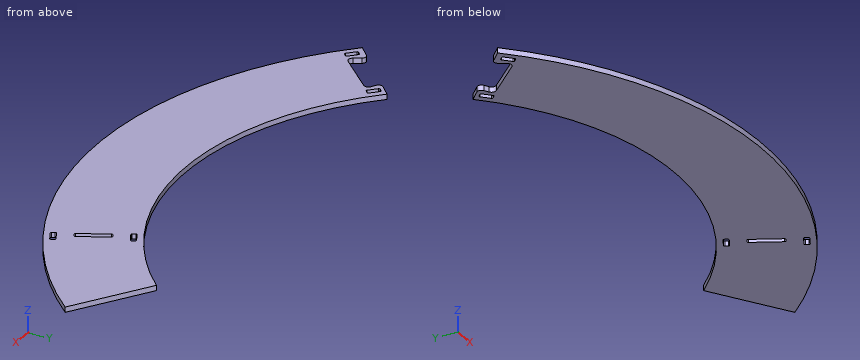
Autodesk Inventor part; units mm, degrees
ref_plane "YZ Plane" through (0, 0, 0) normal (1, 0, 0) x (0, 1, 0)
ref_plane "XZ Plane" through (0, 0, 0) normal (0, 1, 0) x (-1, 0, 0)
ref_plane "XY Plane" through (0, 0, 0) normal (0, 0, 1) x (1, 0, 0)
sketch "CONTOURS" plane through (0, 0, 0) normal (0, 0, 1) x (1, 0, 0)
  arc A0 (18.8569, 427.8827) -> (1891.4893, 468.7097) centre (936.3152, 1313.2613) ccw
  line L0 (18.8569, 427.8827) -> (54.648, 462.3952)
  arc A1 (77.2131, 459.3056) -> (54.648, 462.3952) centre (64.7129, 451.9575) ccw
  line L1 (77.2131, 459.3056) -> (90.7845, 436.2188)
  arc A2 (90.7845, 436.2188) -> (115.4755, 433.495) centre (104.1468, 444.0737) ccw
  line L2 (115.4755, 433.495) -> (224.0619, 549.7797)
  arc A3 (224.0619, 549.7797) -> (220.3778, 573.8421) centre (212.7332, 560.3584) ccw
  line L3 (220.3778, 573.8421) -> (205.6826, 582.1735)
  arc A4 (202.7691, 605.2251) -> (205.6826, 582.1735) centre (212.834, 594.7873) ccw
  line L4 (202.7691, 605.2251) -> (237.5129, 638.7277)
  arc A5 (237.5129, 638.7277) -> (1635.1174, 638.7277) centre (936.3152, 1313.2613) ccw
  line L5 (1635.1174, 638.7277) -> (1891.4893, 468.7097)
sketch "HOLES" plane through (0, 0, 0) normal (0, 0, 1) x (1, 0, 0)
  arc A0 (75.3736, 400.9492) -> (81.0303, 400.9936) centre (78.1798, 403.7997) ccw
  line L0 (75.3736, 400.9492) -> (49.7191, 426.2049)
  arc A1 (49.6748, 431.8616) -> (49.7191, 426.2049) centre (52.5253, 429.0554) ccw
  line L1 (49.6748, 431.8616) -> (57.3918, 439.7004)
  arc A2 (63.0485, 439.7447) -> (57.3918, 439.7004) centre (60.2423, 436.8942) ccw
  line L2 (63.0485, 439.7447) -> (88.703, 414.4891)
  arc A3 (88.7473, 408.8324) -> (88.703, 414.4891) centre (85.8968, 411.6386) ccw
  line L3 (1537.9287, 212.5375) -> (1505.9814, 195.9431)
  arc A4 (1500.5879, 197.6489) -> (1505.9814, 195.9431) centre (1504.1376, 199.4928) ccw
  line L4 (1500.5879, 197.6489) -> (1495.5174, 207.4106)
  arc A5 (1497.2233, 212.8041) -> (1495.5174, 207.4106) centre (1499.0671, 209.2544) ccw
  line L5 (1497.2233, 212.8041) -> (1529.1705, 229.3985)
  arc A6 (1534.564, 227.6927) -> (1529.1705, 229.3985) centre (1531.0143, 225.8489) ccw
  line L6 (1534.564, 227.6927) -> (1539.6345, 217.931)
  arc A7 (1537.9287, 212.5375) -> (1539.6345, 217.931) centre (1536.0848, 216.0872) ccw
  line L7 (1485.873, 267.1962) -> (1476.1114, 262.1257)
  arc A8 (1470.7179, 263.8316) -> (1476.1114, 262.1257) centre (1474.2676, 265.6754) ccw
  line L8 (1470.7179, 263.8316) -> (1420.4735, 360.5606)
  arc A9 (1422.1794, 365.9541) -> (1420.4735, 360.5606) centre (1424.0232, 362.4044) ccw
  line L9 (1422.1794, 365.9541) -> (1431.9411, 371.0247)
  arc A10 (1437.3346, 369.3188) -> (1431.9411, 371.0247) centre (1433.7849, 367.475) ccw
  line L10 (1437.3346, 369.3188) -> (1487.5789, 272.5898)
  arc A11 (1485.873, 267.1962) -> (1487.5789, 272.5898) centre (1484.0292, 270.7459) ccw
  line L11 (1388.5747, 413.294) -> (1383.5041, 423.0556)
  arc A12 (1385.21, 428.4491) -> (1383.5041, 423.0556) centre (1387.0538, 424.8994) ccw
  line L12 (1385.21, 428.4491) -> (1417.1572, 445.0436)
  arc A13 (1422.5507, 443.3377) -> (1417.1572, 445.0436) centre (1419.001, 441.4939) ccw
  line L13 (1422.5507, 443.3377) -> (1427.6212, 433.5761)
  arc A14 (1425.9154, 428.1826) -> (1427.6212, 433.5761) centre (1424.0716, 431.7322) ccw
  line L14 (1425.9154, 428.1826) -> (1393.9682, 411.5881)
  arc A15 (1388.5747, 413.294) -> (1393.9682, 411.5881) centre (1392.1243, 415.1378) ccw
  line L15 (220.1514, 605.0305) -> (227.8684, 612.8694)
  arc A16 (233.5251, 612.9137) -> (227.8684, 612.8694) centre (230.7189, 610.0632) ccw
  line L16 (233.5251, 612.9137) -> (259.1796, 587.658)
  arc A17 (259.2239, 582.0014) -> (259.1796, 587.658) centre (256.3734, 584.8075) ccw
  line L17 (259.2239, 582.0014) -> (251.5069, 574.1625)
  arc A18 (245.8502, 574.1182) -> (251.5069, 574.1625) centre (248.6564, 576.9687) ccw
  line L18 (245.8502, 574.1182) -> (220.1957, 599.3738)
  arc A19 (220.1514, 605.0305) -> (220.1957, 599.3738) centre (223.0019, 602.2243) ccw
  line L19 (543.0858, 821.5545) -> (547.6833, 831.5476)
  arc A20 (547.6833, 831.5476) -> (545.7213, 836.8533) centre (544.0494, 833.2195) ccw
  line L20 (545.7213, 836.8533) -> (513.0165, 851.8999)
  arc A21 (513.0165, 851.8999) -> (507.7108, 849.9379) centre (511.3447, 848.266) ccw
  line L21 (507.7108, 849.9379) -> (503.1133, 839.9447)
  arc A22 (503.1133, 839.9447) -> (505.0753, 834.639) centre (506.7471, 838.2729) ccw
  line L22 (505.0753, 834.639) -> (537.7801, 819.5925)
  arc A23 (537.7801, 819.5925) -> (543.0858, 821.5545) centre (539.4519, 823.2264) ccw
  line L23 (481.0423, 782.4016) -> (435.4847, 683.3788)
  arc A24 (435.4847, 683.3788) -> (437.4468, 678.0731) centre (439.1186, 681.7069) ccw
  line L24 (437.4468, 678.0731) -> (447.4399, 673.4755)
  arc A25 (447.4399, 673.4755) -> (452.7456, 675.4376) centre (449.1117, 677.1094) ccw
  line L25 (452.7456, 675.4376) -> (498.3031, 774.4603)
  arc A26 (498.3031, 774.4603) -> (496.3411, 779.766) centre (494.6693, 776.1322) ccw
  line L26 (496.3411, 779.766) -> (486.348, 784.3636)
  arc A27 (486.348, 784.3636) -> (481.0423, 782.4016) centre (484.6762, 780.7297) ccw
  line L27 (446.1185, 610.7891) -> (441.521, 600.7959)
  arc A28 (436.2153, 598.8339) -> (441.521, 600.7959) centre (437.8871, 602.4678) ccw
  line L28 (436.2153, 598.8339) -> (403.5105, 613.8804)
  arc A29 (401.5485, 619.1861) -> (403.5105, 613.8804) centre (405.1824, 617.5143) ccw
  line L29 (401.5485, 619.1861) -> (406.1461, 629.1793)
  arc A30 (411.4518, 631.1413) -> (406.1461, 629.1793) centre (409.7799, 627.5074) ccw
  line L30 (411.4518, 631.1413) -> (444.1565, 616.0948)
  arc A31 (446.1185, 610.7891) -> (444.1565, 616.0948) centre (442.4847, 612.4609) ccw
  line L31 (88.7473, 408.8324) -> (81.0303, 400.9936)
sketch "LETTERS" plane through (0, 0, 0) normal (0, 0, 1) x (1, 0, 0)
  line L0 (228.3428, 428.6061) -> (222.1589, 433.5761)
  line L1 (222.1589, 433.5761) -> (234.7826, 448.8621)
  line L2 (234.7826, 448.8621) -> (240.0493, 444.5126)
  line L3 (240.0493, 444.5126) -> (240.1714, 444.4197)
  line L4 (240.1714, 444.4197) -> (240.2915, 444.3221)
  line L5 (240.2915, 444.3221) -> (240.4096, 444.2197)
  line L6 (240.4096, 444.2197) -> (240.5256, 444.1125)
  line L7 (240.5256, 444.1125) -> (240.6391, 444.0004)
  line L8 (240.6391, 444.0004) -> (240.7501, 443.8834)
  line L9 (240.7501, 443.8834) -> (240.8585, 443.7615)
  line L10 (240.8585, 443.7615) -> (240.9639, 443.6348)
  line L11 (240.9639, 443.6348) -> (241.0664, 443.5031)
  line L12 (241.0664, 443.5031) -> (241.1657, 443.3666)
  line L13 (228.4677, 428.5172) -> (228.3428, 428.6061)
  line L14 (228.5966, 428.4315) -> (228.4677, 428.5172)
  line L15 (228.7295, 428.3492) -> (228.5966, 428.4315)
  line L16 (228.8663, 428.2704) -> (228.7295, 428.3492)
  line L17 (229.0071, 428.1953) -> (228.8663, 428.2704)
  line L18 (229.1518, 428.1241) -> (229.0071, 428.1953)
  line L19 (229.3004, 428.0569) -> (229.1518, 428.1241)
  line L20 (229.4528, 427.9939) -> (229.3004, 428.0569)
  line L21 (229.609, 427.9352) -> (229.4528, 427.9939)
  line L22 (229.7689, 427.8809) -> (229.609, 427.9352)
  line L23 (229.9324, 427.8313) -> (229.7689, 427.8809)
  line L24 (230.0995, 427.7865) -> (229.9324, 427.8313)
  line L25 (230.2701, 427.7466) -> (230.0995, 427.7865)
  line L26 (230.444, 427.7117) -> (230.2701, 427.7466)
  line L27 (230.6212, 427.6819) -> (230.444, 427.7117)
  line L28 (230.8016, 427.6574) -> (230.6212, 427.6819)
  line L29 (230.9849, 427.6383) -> (230.8016, 427.6574)
  line L30 (231.1712, 427.6246) -> (230.9849, 427.6383)
  line L31 (231.3602, 427.6165) -> (231.1712, 427.6246)
  line L32 (231.5519, 427.6141) -> (231.3602, 427.6165)
  line L33 (231.7459, 427.6174) -> (231.5519, 427.6141)
  line L34 (231.9423, 427.6264) -> (231.7459, 427.6174)
  line L35 (232.1408, 427.6413) -> (231.9423, 427.6264)
  line L36 (232.3412, 427.662) -> (232.1408, 427.6413)
  line L37 (232.5433, 427.6887) -> (232.3412, 427.662)
  line L38 (232.747, 427.7212) -> (232.5433, 427.6887)
  line L39 (232.9521, 427.7597) -> (232.747, 427.7212)
  line L40 (233.1584, 427.8041) -> (232.9521, 427.7597)
  line L41 (233.3656, 427.8544) -> (233.1584, 427.8041)
  line L42 (233.5736, 427.9106) -> (233.3656, 427.8544)
  line L43 (233.7821, 427.9726) -> (233.5736, 427.9106)
  line L44 (233.991, 428.0404) -> (233.7821, 427.9726)
  line L45 (234.2, 428.1139) -> (233.991, 428.0404)
  line L46 (234.409, 428.193) -> (234.2, 428.1139)
  line L47 (234.6177, 428.2776) -> (234.409, 428.193)
  line L48 (234.8258, 428.3677) -> (234.6177, 428.2776)
  line L49 (235.0333, 428.4632) -> (234.8258, 428.3677)
  line L50 (235.2399, 428.5638) -> (235.0333, 428.4632)
  line L51 (235.4454, 428.6696) -> (235.2399, 428.5638)
  line L52 (235.6496, 428.7803) -> (235.4454, 428.6696)
  line L53 (235.8522, 428.8958) -> (235.6496, 428.7803)
  line L54 (236.0532, 429.0159) -> (235.8522, 428.8958)
  line L55 (236.2524, 429.1405) -> (236.0532, 429.0159)
  line L56 (236.4495, 429.2695) -> (236.2524, 429.1405)
  line L57 (236.6444, 429.4026) -> (236.4495, 429.2695)
  line L58 (236.8369, 429.5396) -> (236.6444, 429.4026)
  line L59 (237.0269, 429.6804) -> (236.8369, 429.5396)
  line L60 (237.2142, 429.8249) -> (237.0269, 429.6804)
  line L61 (237.3987, 429.9727) -> (237.2142, 429.8249)
  line L62 (237.5803, 430.1237) -> (237.3987, 429.9727)
  line L63 (237.7587, 430.2777) -> (237.5803, 430.1237)
  line L64 (237.934, 430.4346) -> (237.7587, 430.2777)
  line L65 (238.2747, 430.7559) -> (237.934, 430.4346)
  line L66 (238.6014, 431.0861) -> (238.2747, 430.7559)
  line L67 (238.9137, 431.4236) -> (238.6014, 431.0861)
  line L68 (239.2109, 431.7669) -> (238.9137, 431.4236)
  line L69 (239.4929, 432.1144) -> (239.2109, 431.7669)
  line L70 (239.7594, 432.4649) -> (239.4929, 432.1144)
  line L71 (240.0148, 432.8236) -> (239.7594, 432.4649)
  line L72 (240.2628, 433.1961) -> (240.0148, 432.8236)
  line L73 (240.5022, 433.582) -> (240.2628, 433.1961)
  line L74 (240.7316, 433.9805) -> (240.5022, 433.582)
  line L75 (240.9497, 434.3906) -> (240.7316, 433.9805)
  line L76 (241.1552, 434.8114) -> (240.9497, 434.3906)
  line L77 (241.2528, 435.0254) -> (241.1552, 434.8114)
  line L78 (241.3468, 435.2416) -> (241.2528, 435.0254)
  line L79 (241.4371, 435.4598) -> (241.3468, 435.2416)
  line L80 (241.5233, 435.68) -> (241.4371, 435.4598)
  line L81 (241.6055, 435.9017) -> (241.5233, 435.68)
  line L82 (241.6835, 436.125) -> (241.6055, 435.9017)
  line L83 (241.7571, 436.3496) -> (241.6835, 436.125)
  line L84 (241.8262, 436.5752) -> (241.7571, 436.3496)
  line L85 (241.8908, 436.8018) -> (241.8262, 436.5752)
  line L86 (241.9505, 437.0289) -> (241.8908, 436.8018)
  line L87 (242.0055, 437.2566) -> (241.9505, 437.0289)
  line L88 (242.0555, 437.4844) -> (242.0055, 437.2566)
  line L89 (242.1005, 437.7123) -> (242.0555, 437.4844)
  line L90 (242.1404, 437.9399) -> (242.1005, 437.7123)
  line L91 (242.175, 438.1671) -> (242.1404, 437.9399)
  line L92 (242.2045, 438.3936) -> (242.175, 438.1671)
  line L93 (242.2286, 438.6191) -> (242.2045, 438.3936)
  line L94 (242.2474, 438.8435) -> (242.2286, 438.6191)
  line L95 (242.2608, 439.0665) -> (242.2474, 438.8435)
  line L96 (242.2688, 439.288) -> (242.2608, 439.0665)
  line L97 (242.2714, 439.5075) -> (242.2688, 439.288)
  line L98 (242.2686, 439.7251) -> (242.2714, 439.5075)
  line L99 (242.2604, 439.9404) -> (242.2686, 439.7251)
  line L100 (242.2468, 440.1532) -> (242.2604, 439.9404)
  line L101 (242.2279, 440.3633) -> (242.2468, 440.1532)
  line L102 (242.2037, 440.5706) -> (242.2279, 440.3633)
  line L103 (242.1742, 440.7747) -> (242.2037, 440.5706)
  line L104 (242.1395, 440.9757) -> (242.1742, 440.7747)
  line L105 (242.0998, 441.1732) -> (242.1395, 440.9757)
  line L106 (242.055, 441.3671) -> (242.0998, 441.1732)
  line L107 (242.0052, 441.5573) -> (242.055, 441.3671)
  line L108 (241.9506, 441.7435) -> (242.0052, 441.5573)
  line L109 (241.8913, 441.9258) -> (241.9506, 441.7435)
  line L110 (241.8274, 442.1039) -> (241.8913, 441.9258)
  line L111 (241.759, 442.2776) -> (241.8274, 442.1039)
  line L112 (241.6862, 442.447) -> (241.759, 442.2776)
  line L113 (241.6092, 442.612) -> (241.6862, 442.447)
  line L114 (241.5281, 442.7723) -> (241.6092, 442.612)
  line L115 (241.443, 442.928) -> (241.5281, 442.7723)
  line L116 (241.3542, 443.079) -> (241.443, 442.928)
  line L117 (241.2617, 443.2252) -> (241.3542, 443.079)
  line L118 (241.1657, 443.3666) -> (241.2617, 443.2252)
extrude "Extrusion4" add sketch "CONTOURS" along normal blind 18
extrude "Extrusion5" cut sketch "HOLES" along normal blind 18 contours L0 A1 L1 A2 L2 A3 L31 A0 | L3 A4 L4 A5 L5 A6 L6 A7 | L7 A8 L8 A9 L9 A10 L10 A11 | L11 A12 L12 A13 L13 A14 L14 A15 | L15 A16 L16 A17 L17 A18 L18 A19
properties part number "Platform D4" material "Wood (Birch)"
The model under review builds one solid part; all positions refer to its coordinate system, in mm. Coordinates: 2 decimals unless noted, no trailing zeros. Loops run counter-clockwise (first coordinate to the right, second up) from the corner with the lowest first, then second, coordinate; pieces in that order, holes last. Notation, with made-up numbers: M 66,-22 L 106,-22 A15 cw 106,-13 Z; hole C 41.5,85.25 d9. An arc over 180 degrees is marked long. Put each result on its own line as item: value. Start each with the question number.
Q1. Add section C-C (y = 324.5). Write out the cut boundary in (x, z) (3 decimals).
Q2. Wall thickness on line 1 (X direction, y = 590, z = 14.25); line 2 (X direction, y = 414.5, z = 1.75); line 3 (X direction, y = 431, z = 10): over which ranges is each line inside the solid? List them lowest first.
Q3. Add section D-D (x = 1706). Write out the cut boundary in (y, z).
Q4. Add section B-B (z = 11.5). Count the separate pieces of the cut face and the enclosed holes in it, and give its area (3 significant figures).
Q5. Clearance check with flat-ended pins moving along their axes: pin 1 (8 mm diameter, centred on y = 259, z = 15, fed in from -X); pin 2 (10 mm diameter, centred on y = 521.5, z = 11.5, fed in from +X); pin 3 (10 mm diameter, centred on x = 1358, z = 9, fed in from +Y); pin 4 (4 mm diameter, centred on x = 274.5, y = 416.5, fed in from -Z). State where each tip first meets the part, or that it passes through.
Q6. Add section A-A (y = 523.5). Write out the cut boundary in (x, z).
Answers:
1. outline: M 131.346,0 L 1439.205,0 L 1439.205,18 L 131.346,18 Z; M 1460.615,0 L 1741.285,0 L 1741.285,18 L 1460.615,18 Z
2. line 1: x = 199.15 to 229.72, 256.8 to 288.08, 1584.55 to 1708.59
2. line 2: x = 31.96 to 61.61, 88.69 to 568.15, 1304.48 to 1387.95, 1399.57 to 1840.67
2. line 3: x = 22.09 to 49.03, 71.93 to 95.82, 112.47 to 530.19, 1342.44 to 1390.12, 1428 to 1856.77
3. outline: M 296.79,0 L 591.72,0 L 591.72,18 L 296.79,18 Z
4. separate pieces: 1
4. enclosed holes: 5
4. area: 540,000 mm^2
5. pin 1: stops at x = 213.42
5. pin 2: stops at x = 1819.43
5. pin 3: stops at y = 440.76
5. pin 4: stops at z = 0
6. outline: M 199.52,0 L 370.99,0 L 370.99,18 L 199.52,18 Z; M 1501.64,0 L 1808.87,0 L 1808.87,18 L 1501.64,18 Z
